Check sheet for the modelled part. Datum: model origin and axes. Units: mm. Face numbers are marked on the shaded views. Coordinates: 2 decimals unless noted, no trailing zeros. Loops run counter-clockwise (first coordinate to the right, second up) from the corner with the lowest first, then second, coordinate; pieces in that order, holes last.
```python
from build123d import *

# Parameters (mm, degrees)
F0_R     = 20
F1_DEPTH = 50
F2_R     = 12.7
F3_DEPTH = 43
F4_SIZE  = 1


with BuildPart() as f1:
    # F0 (on Top) → F1 (new body)
    with BuildSketch(Plane.XY):
        Circle(F0_R)
    extrude(amount=F1_DEPTH)

    # F2 (on face) → F3 (cut)
    with BuildSketch(Plane(origin=(0, 0, 0), x_dir=(1, 0, 0), z_dir=(0, 0, -1))):
        Circle(F2_R)
    extrude(amount=-F3_DEPTH, mode=Mode.SUBTRACT)

    # F4
    f4_edges = [f1.edges().sort_by_distance(p)[0] for p in [
        (-12.7, 0, 0),
        (-20, 0, 0),
        (-20, 0, 50),
    ]]
    chamfer(f4_edges, length=F4_SIZE)


solid = f1.part
```
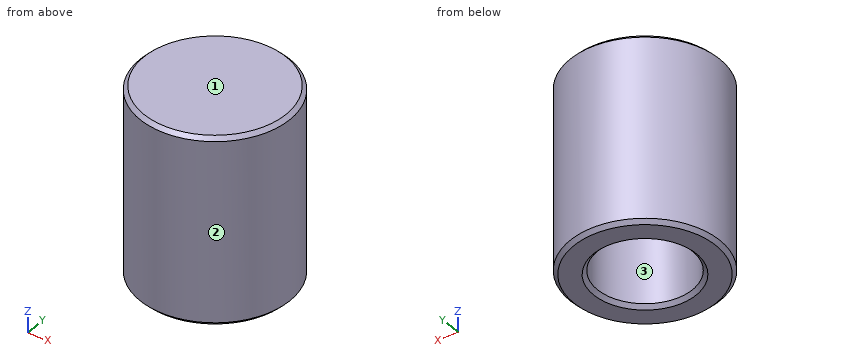
1) Depth check by flat-ended pin: pin 1 (2 mm diameter, centred on y = 6, z = 44.5, fed in from +X); pin 2 (8 mm diameter, centred on x = 0, z = 29, fed in from -Y); pin 3 (1.5 mm diameter, centred on x = -12.5, y = 16, fed in from -Z). Enter the tip coordinate at first touch or a pass-through.
Answer sheet:
pin 1: stops at x = 19.36
pin 2: stops at y = -20
pin 3: stops at z = 0.55
2) Section check B-B on z = 15.5. Enter the section's corners in (x, y).
Answer sheet:
outline: circle Ø40 at (0, 0); hole circle Ø25.4 at (0, 0)
3) Section check A-A on x = 0. Enter the section's corners in (y, z).
Answer sheet:
outline: (-20, 1) - (-19, 0) - (-13.7, 0) - (-12.7, 1) - (-12.7, 43) - (12.7, 43) - (12.7, 1) - (13.7, 0) - (19, 0) - (20, 1) - (20, 49) - (19, 50) - (-19, 50) - (-20, 49) - close
4) Scan lines: line 1 (Y direction, x = 0, z = 12); line 2 (Y direction, x = -9.5, z = 15); line 3 (X direction, y = 3.5, z = 10.5). Record each from-to range of solid material in increasing order.
Answer sheet:
line 1: y = -20 to -12.7, 12.7 to 20
line 2: y = -17.6 to -8.43, 8.43 to 17.6
line 3: x = -19.69 to -12.21, 12.21 to 19.69
5) Mould release check, pull along X, two halves, no side actions. Record for the marked faces 1, 2 and 3: +X half, -X half, draft (parallel to the pull), parting line (faces both ways), or undercut.
Answer sheet:
face 1: draft
face 2: parting line
face 3: undercut
6) Section check D-D on z = 46. Enter the section's corners in (x, y).
Answer sheet:
outline: circle Ø40 at (0, 0)
